Geometry check sheet. Reference: the model listing, model coordinates, mm. A direction names the side the tool comes from. Give positions to 0.01 mm unless a question says otherwise; leave off trailing zeros. Loops run counter-clockwise (first coordinate to the right, second up) from the corner with the lowest first, then second, coordinate; pieces in that order, holes last.
1. Cross-section at A-A, the plane y = 0. Record the cut outline in (x, z).
2. Release check for a two-part mould opening along Y. For faces 1 (the flat face through (10, -8, -0.75)), 2 (the conical face through (-7.67, -3.1, 0.69)), 3 (the cylindrical face through (7.395, 3.408, -8.219)), 4 (the flat face through (14, 11, 2.5)) record: +Y half, -Y half, draft (parallel to the pull), parting line (faces both ways), or undercut.
3. Cross-section at B-B, the plane z = 0. Record the cut outline in (x, y), plus the area to 3 significant figures.
4. Go/stop test with flat-tipped pins: pin 1 Ø0.6 at (x, y) = (14.5, 10.5) entering from -Z; pin 2 Ø2 at (x, y) = (8, -8) entering from -Z; pin 3 Ø1 at (x, z) = (-6.5, -4) entering from +Y; pin 4 Ø1 at (y, z) = (8, 0) entering from +X. Record where each tip stops, or that it passes through.
5. Tool access check on faces 5 (the cylindrical face through (7.395, -6.237, -3.977)), 6 (the flat face through (14, 13.897, 0)), 7 (the flat face through (14, 11, -2.5)). Record the directions out of +Z, -Z, +X, -X, +Y, -Y that give a thin tool (end or side, any length) a straight path to the whole face; none if there is none.
6. Cross-section at D-D, the plane x = 1.5. Record the cut outline in (y, z).
7. Cross-section at C-C, the plane x = 10.5. Record the cut outline in (y, z).
8. Material ranges on L1, parallel to Z at x = 4.5, y = 0; L2, parallel to Y at x = 8, z = 0; L3, parallel to Y at x = -8, z = -2.75, recorded low to high.
Autodesk Inventor part; units mm, degrees
ref_plane "YZ Plane" through (0, 0, 0) normal (1, 0, 0) x (0, 1, 0)
ref_plane "XZ Plane" through (0, 0, 0) normal (0, 1, 0) x (-1, 0, 0)
ref_plane "XY Plane" through (0, 0, 0) normal (0, 0, 1) x (1, 0, 0)
sketch "Sketch1" plane through (0, 0, 0) normal (0, 1, 0) x (-1, 0, 0)
  line L0 (0, 0) -> (12.5354, 0)
  line L1 (12.5354, 0) -> (12.5354, -2)
  line L2 (12.5354, -2) -> (0, -8.897)
  line L3 (0, -8.897) -> (0, -7.397)
  line L4 (10.9043, 0) -> (10.9043, -1.3974)
  line L5 (0, -7.397) -> (10.9043, -1.3974)
  dimension "d0" = 2
  dimension "d23" = 1.5
revolve "Revolution1" add sketch "Sketch1" angle 360 about axis through (0, 0, 0) along (-1, 0, 0)
sketch "Sketch2" plane through (0, 0, 0) normal (1, 0, 0) x (0, 0, -1)
  point P0 (0, 0)
sketch "Sketch3" plane through (-12.5354, 0, 0) normal (-1, 0, 0) x (0, 0, 1)
  point P0 (0, 0)
sketch "Sketch4" plane through (-12.5354, 0, 0) normal (-1, 0, 0) x (0, 0, 1)
  circle A0 centre (0, 0) radius 1.5
  dimension "d37" = 3
sketch "Sketch5" plane through (-12.5354, 0, 0) normal (-1, 0, 0) x (0, 0, 1)
  point P0 (0, 0)
extrude "Extrusion1" cut sketch "Sketch4" against normal blind 10
sketch "Sketch6" plane through (-2.3704, 0, 0) normal (-1, 0, 0) x (0, 0, 1)
  circle A0 centre (0, 0) radius 2
sketch "Sketch7" plane through (0, 0, 0) normal (1, 0, 0) x (0, 0, -1)
  circle A0 centre (0, 0) radius 8.897
extrude "Extrusion2" [suppressed]
sketch "Sketch8" plane through (15, 0, 0) normal (1, 0, 0) x (0, 0, -1)
  circle A0 centre (0, 0) radius 8.897
  line L0 (-8.6693, -2) -> (-13.1693, -2)
  line L1 (-13.1693, -2) -> (-13.1693, 0)
  line L2 (-13.1693, 0) -> (-8.897, 0)
  line L3 (-8.6693, 2) -> (-13.1693, 2)
  line L4 (-13.1693, 2) -> (-13.1693, 0)
  line L5 (0, -8.897) -> (0, 8.897)
  line L6 (8.6693, -2) -> (13.1693, -2)
  line L7 (13.1693, -2) -> (13.1693, 0)
  line L8 (13.1693, 0) -> (8.897, 0)
  line L9 (8.6693, 2) -> (13.1693, 2)
  line L10 (13.1693, 2) -> (13.1693, 0)
  dimension "d8" = 4.5
  dimension "d9" = 2
extrude "Extrusion3" [suppressed]
sketch "Sketch9" plane through (15, 0, 0) normal (1, 0, 0) x (0, 0, -1)
  point P0 (0, 0)
sketch "Sketch10" plane through (15, 0, 0) normal (1, 0, 0) x (0, 0, -1)
  point P0 (0, 0)
sketch "Sketch11" plane through (15, 0, 0) normal (1, 0, 0) x (0, 0, -1)
  point P0 (0, 0)
sketch "Sketch12" plane through (15, 0, 0) normal (1, 0, 0) x (0, 0, -1)
  circle A0 centre (0, 0) radius 7.5
  dimension "d12" = 15
sketch "Sketch13" plane through (15, 0, 0) normal (1, 0, 0) x (0, 0, -1)
  line L0 (6.4465, 0.75) -> (8.4465, 0.75)
  line L1 (8.4465, 0.75) -> (8.4465, -0.75)
  line L2 (8.4465, -0.75) -> (6.4465, -0.75)
  line L3 (6.4465, -0.75) -> (6.4465, 0.75)
  line L4 (6.4465, 0.75) -> (8.4465, -0.75) construction
  line L5 (8.4465, 0.75) -> (6.4465, -0.75) construction
  line L6 (0, 7.445) -> (0, -3.9697)
  line L7 (-6.4465, 0.75) -> (-8.4465, 0.75)
  line L8 (-8.4465, 0.75) -> (-8.4465, -0.75)
  line L9 (-8.4465, -0.75) -> (-6.4465, -0.75)
  line L10 (-6.4465, -0.75) -> (-6.4465, 0.75)
  line L11 (-6.4465, 0.75) -> (-8.4465, -0.75) construction
  line L12 (-8.4465, 0.75) -> (-6.4465, -0.75) construction
  point P0 (0, 0)
  point P1 (7.4465, 0)
  point P2 (-7.4465, 0)
  dimension "d13" = 2
  dimension "d14" = 1.5
extrude "Extrusion4" [suppressed]
extrude "Extrusion5" [suppressed]
extrude "Extrusion6" [suppressed]
sketch "Sketch14" plane through (-2.3704, 0, 0) normal (-1, 0, 0) x (0, 0, 1)
  circle A0 centre (0, 0) radius 2
extrude "Extrusion7" [suppressed]
sketch "Sketch15" plane through (0, 0, 0) normal (1, 0, 0) x (0, 0, -1)
  circle A0 centre (0, 0) radius 8.897
  circle A1 centre (0, 0) radius 7.397
extrude "Extrusion8" add sketch "Sketch15" along normal blind 15
sketch "Sketch16" plane through (15, 0, 0) normal (1, 0, 0) x (0, 0, -1)
  point P0 (0, 0)
sketch "Sketch17" plane through (15, 0, 0) normal (1, 0, 0) x (0, 0, -1)
  circle A0 centre (0, 0) radius 8.897
  line L0 (0, 8.897) -> (0, 13.897)
  line L1 (0, 13.897) -> (-2.5, 13.897)
  line L2 (-2.5, 13.897) -> (-2.5, 8.5385)
  line L3 (0, 13.897) -> (2.5, 13.897)
  line L4 (2.5, 13.897) -> (2.5, 8.5385)
  line L5 (-7.2862, 0) -> (2, 0)
  circle A1 centre (0, 0) radius 2
  line L6 (0, -8.897) -> (0, -13.897)
  line L7 (0, -13.897) -> (-2.5, -13.897)
  line L8 (-2.5, -13.897) -> (-2.5, -8.5385)
  line L9 (0, -13.897) -> (2.5, -13.897)
  line L10 (2.5, -13.897) -> (2.5, -8.5385)
  dimension "d29" = 5
  dimension "d30" = 2.5
extrude "Extrusion9" add sketch "Sketch17" against normal blind 2 contours A0 L0 L3 L4 | L10 L9 L6 A0 | A0 L2 L1 L0 | L6 L7 L8 A0
sketch "Sketch18" plane through (15, 0, 0) normal (1, 0, 0) x (0, 0, -1)
  circle A0 centre (0, 0) radius 7.397
  line L0 (0, -7.397) -> (0, -8.297)
  line L1 (0, -8.297) -> (-0.75, -8.297)
  line L2 (-0.75, -8.297) -> (-0.75, -7.3588)
  line L3 (0, -8.297) -> (0.75, -8.297)
  line L4 (0.75, -8.297) -> (0.75, -7.3588)
  line L5 (-4.4895, 0) -> (3.1188, 0)
  line L6 (0, 7.397) -> (0, 8.297)
  line L7 (0, 8.297) -> (-0.75, 8.297)
  line L8 (-0.75, 8.297) -> (-0.75, 7.3588)
  line L9 (0, 8.297) -> (0.75, 8.297)
  line L10 (0.75, 8.297) -> (0.75, 7.3588)
  dimension "d33" = 0.9
  dimension "d34" = 0.75
extrude "Extrusion10" cut sketch "Sketch18" against normal blind 10 contours A0 L6 L9 L10 | L4 L3 L0 A0 | A0 L8 L7 L6 | L0 L1 L2 A0
sketch "Sketch19" plane through (15, 0, 0) normal (1, 0, 0) x (0, 0, -1)
  point P0 (0, 0)
thread "Thread3"
properties part number "Joy stick part 2"
Result:
1. outline: (-12.54, -2) - (0, -8.9) - (15, -8.9) - (15, -7.4) - (0, -7.4) - (-10.72, -1.5) - (-12.54, -1.5) - close; (-12.54, 1.5) - (-10.72, 1.5) - (0, 7.4) - (15, 7.4) - (15, 8.9) - (0, 8.9) - (-12.54, 2) - close
2. face 1: undercut
2. face 2: undercut
2. face 3: parting line
2. face 4: draft
3. outline: (-12.54, -2) - (0, -8.9) - (13, -8.9) - (13, -13.9) - (15, -13.9) - (15, -8.3) - (5, -8.3) - (5, -7.4) - (0, -7.4) - (-10.72, -1.5) - (-12.54, -1.5) - close; (-12.54, 1.5) - (-10.72, 1.5) - (0, 7.4) - (5, 7.4) - (5, 8.3) - (15, 8.3) - (15, 13.9) - (13, 13.9) - (13, 8.9) - (0, 8.9) - (-12.54, 2) - close
3. area: 82.8 mm2
4. pin 1: stops at z = -2.5
4. pin 2: stops at z = -5.49
4. pin 3: stops at y = 4.14
4. pin 4: stops at x = 15
5. face 5: +X
5. face 6: +Z, -Z, +X, -X, +Y
5. face 7: -Z, +X, -X, +Y
6. outline: circle Ø17.79 at (0, 0); hole circle Ø14.79 at (0, 0)
7. outline: circle Ø17.79 at (0, 0); hole (-8.3, -0.75) - (-7.36, -0.75) arc R7.4 ccw to (7.36, -0.75) - (8.3, -0.75) - (8.3, 0.75) - (7.36, 0.75) arc R7.4 ccw to (-7.36, 0.75) - (-8.3, 0.75) - close
8. L1: z = -8.9 to -7.4, 7.4 to 8.9
8. L2: y = -8.9 to -8.3, 8.3 to 8.9
8. L3: y = -3.56 to -1.19, 1.19 to 3.56
